```python
from build123d import *

# Parameters (mm, degrees)
F1_DEPTH       = 82.55
F2_DEPTH       = 12.7
F4_D           = 10.414
F4_CBORE_D     = 17.526
F4_CBORE_DEPTH = 9.906
F6_D           = 10.414
F6_CBORE_D     = 17.526
F6_CBORE_DEPTH = 9.906
F7_W           = 38.1
F7_H           = 69.85
F8_DEPTH       = 25.4
F9_SIZE        = 2.032
F10_SIZE       = 2.032
F11_SIZE       = 2.032
F12_SIZE       = 2.032
F13_SIZE       = 2.032
F14_SIZE       = 2.032


with BuildPart() as f1:
    # F0 (on Top) → F1 (new body)
    with BuildSketch(Plane.XY):
        Polygon((-72.4953562021, 0), (0, 0), (0, 76.2), (-25.4, 76.2), (-25.4, 25.4), (-63.5, 25.4), (-76.2, 25.4), (-76.2, 0), align=None)
    extrude(amount=F1_DEPTH)

    # F0 (on Top) → F2 (join)
    with BuildSketch(Plane.XY):
        Polygon((-72.4953562021, 0), (0, 0), (0, 76.2), (-25.4, 76.2), (-25.4, 25.4), (-63.5, 25.4), (-76.2, 25.4), (-76.2, 0), align=None)
        with BuildLine():
            Line((-25.4, 76.2), (0, 76.2))
            Line((0, 76.2), (0, 88.9))
            ThreePointArc((0, 88.9), (-3.7197438789, 97.8802561211), (-12.7, 101.6))
            ThreePointArc((-12.7, 101.6), (-21.6802561211, 97.8802561211), (-25.4, 88.9))
            Line((-25.4, 88.9), (-25.4, 76.2))
        make_face()
        with BuildLine():
            Line((-88.9, 0), (-76.2, 0))
            Line((-76.2, 0), (-76.2, 25.4))
            Line((-76.2, 25.4), (-88.9, 25.4))
            ThreePointArc((-88.9, 25.4), (-97.8802561211, 21.6802561211), (-101.6, 12.7))
            ThreePointArc((-101.6, 12.7), (-97.8802561211, 3.7197438789), (-88.9, 0))
        make_face()
    extrude(amount=F2_DEPTH)

    # F4 (through all)
    with Locations(Plane.XY.offset(12.7)):
        with Locations((-12.7, 88.9)):
            CounterBoreHole(F4_D / 2, F4_CBORE_D / 2, F4_CBORE_DEPTH)

    # F6 (through all)
    with Locations(Plane.XY.offset(12.7)):
        with Locations((-88.9, 12.7)):
            CounterBoreHole(F6_D / 2, F6_CBORE_D / 2, F6_CBORE_DEPTH)

    # F7 (on face) → F8 (cut)
    with BuildSketch(Plane(origin=(0, 25.4, 0), x_dir=(-1, 0, 0), z_dir=(0, 1, 0))):
        with Locations((44.45, 34.925)):
            Rectangle(F7_W, F7_H)
    extrude(amount=-F8_DEPTH, mode=Mode.SUBTRACT)

    # F9
    f9_edges = [f1.edges().sort_by_distance(p)[0] for p in [
        (0, 38.1, 82.55),
    ]]
    chamfer(f9_edges, length=F9_SIZE)

    # F10
    f10_edges = [f1.edges().sort_by_distance(p)[0] for p in [
        (-39.116, 0, 82.55),
    ]]
    chamfer(f10_edges, length=F10_SIZE)

    # F11
    f11_edges = [f1.edges().sort_by_distance(p)[0] for p in [
        (-25.4, 50.8, 82.55),
    ]]
    chamfer(f11_edges, length=F11_SIZE)

    # F12
    f12_edges = [f1.edges().sort_by_distance(p)[0] for p in [
        (-50.8, 25.4, 82.55),
    ]]
    chamfer(f12_edges, length=F12_SIZE)

    # F13
    f13_edges = [f1.edges().sort_by_distance(p)[0] for p in [
        (-12.7, 76.2, 82.55),
    ]]
    chamfer(f13_edges, length=F13_SIZE)

    # F14
    f14_edges = [f1.edges().sort_by_distance(p)[0] for p in [
        (-76.2, 12.7, 82.55),
    ]]
    chamfer(f14_edges, length=F14_SIZE)


solid = f1.part
```
Can you work these out from the model? Positions are in its coordinate system, mm. A direction names the side the tool comes from. Give positions to 0.01 mm unless a question says otherwise; leave off trailing zeros. Order: outer loops, then holes, each group sorted by start corner. A loop starts at its lowest first (then second) coordinate and runs counter-clockwise, first axis right, second up. Notation, with made-up numbers: (17, 58) - (35, 58) arc R19 cw to (35, 94) - close; hole circle Ø4 at (56, -33). An arc over 180 degrees is marked (long way). Use a Markdown table: item, result. Add a question column.
Q1. If we mould it in two halves opening along Y, with no side actions, what happens to faces 1 (the flat face through (-25, 0, 40)), 2 (the cylindrical face through (-83.7, 12.93, 1.38)), 3 (the flat face through (0, 44, 40)), 4 (the flat face through (-13, 76.2, 46))? For each: released by +Y, released by -Y, zero draft, split by the parting line, or undercut.
Q2. If we section it at D-D on x = -40: Write out the boundary of the cut face in (y, z), plus the area to 3 significant figures.
Q3. On a 3-axis mill with a long thin cutter (end or side, diameter ignored), from which of +Z, -Z, +X, -X, +Y, -Y can I reach the whole of each face in a straight line? I mean faces 5 (the cylindrical face through (-13.84, 97.59, 7.82)), 6 (the flat face through (-76.2, 13, 46)), 7 (the flat face through (-21.3, 86.3, 12.7)), 8 (the flat face through (-64, 25.4, 49)). Say none if no direction works.
Q4. If we section it at A-A on z = 10.5: Write out the boundary of the cut face in (x, y), plus the area to 3 significant figures.
Q5. If we section it at B-B on z = 56.5: Write out the boundary of the cut face in (x, y), plus the area to 3 significant figures.
Q6. If we section it at C-C on y = 16.5: Write out the boundary of the cut face in (x, z), plus the area to 3 significant figures.
Q7. Please list where these lines run through material, in increasing order: line 1 along X through (y, z) = (52, 44.5); line 2 along Z through (x, y) = (-59, 23); line 3 along X through (y, z) = (24, 27).
Q8. I'm going to push flat-ended pins straight in: pin 1 (7.5 mm diameter, centred on x = -46, y = 17, fed in from -Z); pin 2 (12.5 mm diameter, centred on x = -16, y = 87.5, fed in from +Z); pin 3 (13.5 mm diameter, centred on x = -12.7, y = 88.9, fed in from +Z). Where does each tip first touch, or does it pass through?
Answers follow:
| question | item | result |
|---|---|---|
| 1 | face 1 | released by -Y |
| 1 | face 2 | undercut |
| 1 | face 3 | zero draft |
| 1 | face 4 | released by +Y |
| 2 | outline | (0, 69.85) - (25.4, 69.85) - (25.4, 80.52) - (23.37, 82.55) - (2.03, 82.55) - (0, 80.52) - close |
| 2 | area | 318 mm^2 |
| 3 | face 5 | +Z |
| 3 | face 6 | +Z, -X, +Y, -Y |
| 3 | face 7 | +Z, +X, -X, +Y |
| 3 | face 8 | +Z, -Z, -X, +Y |
| 4 | outline | (-88.9, 0) - (-63.5, 0) - (-63.5, 25.4) - (-88.9, 25.4) arc R12.7 ccw to start; (-25.4, 0) - (0, 0) - (0, 88.9) arc R12.7 ccw to (-25.4, 88.9) - close; hole circle Ø17.53 at (-88.9, 12.7); hole circle Ø17.53 at (-12.7, 88.9) |
| 4 | area | 2,930 mm^2 |
| 5 | outline | (-76.2, 0) - (-63.5, 0) - (-63.5, 25.4) - (-76.2, 25.4) - close; (-25.4, 0) - (0, 0) - (0, 76.2) - (-25.4, 76.2) - close |
| 5 | area | 2,260 mm^2 |
| 6 | outline | (-101.02, 0) - (-92.46, 0) - (-92.46, 2.79) - (-96.8, 2.79) - (-96.8, 12.7) - (-101.02, 12.7) - close; (-85.34, 0) - (-63.5, 0) - (-63.5, 69.85) - (-25.4, 69.85) - (-25.4, 0) - (0, 0) - (0, 80.52) - (-2.03, 82.55) - (-74.17, 82.55) - (-76.2, 80.52) - (-76.2, 12.7) - (-81, 12.7) - (-81, 2.79) - (-85.34, 2.79) - close |
| 6 | area | 3,760 mm^2 |
| 7 | line 1 | x = -25.4 to 0 |
| 7 | line 2 | z = 69.85 to 82.55 |
| 7 | line 3 | x = -76.2 to -63.5, -25.4 to 0 |
| 8 | pin 1 | stops at z = 69.85 |
| 8 | pin 2 | stops at z = 12.7 |
| 8 | pin 3 | stops at z = 2.79 |
